```python
from build123d import *

# Parameters (mm, degrees)
SKETCH1_W           = 12.94
SKETCH1_H           = 7.76
BOSS_EXTRUDE1_DEPTH = 9.46
SKETCH2_R           = 2.87
BOSS_EXTRUDE2_DEPTH = 8.11
SKETCH4_W           = 0.73
SKETCH4_H           = 2.27
BOSS_EXTRUDE3_DEPTH = 4.33
BOSS_EXTRUDE4_DEPTH = 1.68
SKETCH6_R           = 6
BOSS_EXTRUDE5_DEPTH = 1.7
BOSS_EXTRUDE6_DEPTH = 1.68


with BuildPart() as part:
    # Sketch1 → Boss-Extrude1 (new body)
    with BuildSketch(Plane.XY):
        Rectangle(SKETCH1_W, SKETCH1_H)
    extrude(amount=BOSS_EXTRUDE1_DEPTH)

    # Sketch2 → Boss-Extrude2 (add)
    with BuildSketch(Plane.XY.offset(9.46)):
        Circle(SKETCH2_R)
    extrude(amount=BOSS_EXTRUDE2_DEPTH)

    # Sketch3 → Revolve1 (revolve)
    with BuildSketch(Plane(origin=(0, 0, 0), x_dir=(1, 0, 0), z_dir=(0, 1, 0))):
        with BuildLine():
            Line((0.46866366, -17.57), (-2.564053278, -27.111612822))
            ThreePointArc((-2.564053278, -27.111612822), (-3.316297804, -27.98726181), (-4.468815416, -28.053111116))
            Line((-4.468815416, -28.053111116), (-0.702418437, -17.57))
            Line((-0.702418437, -17.57), (0.46866366, -17.57))
        make_face()
    revolve(axis=Axis((-4.468815416, 0, 28.053111116), (0.3381215193488044, 0, -0.9411024589029912)))

    # Sketch4 → Boss-Extrude3 (add)
    with BuildSketch(Plane(origin=(0, 0, 0), x_dir=(-1, 0, 0), z_dir=(0, 0, -1))):
        Rectangle(SKETCH4_W, SKETCH4_H)
        with Locations((-4.475, 0)):
            Rectangle(SKETCH4_W, SKETCH4_H)
        with Locations((4.475, 0)):
            Rectangle(SKETCH4_W, SKETCH4_H)
    extrude(amount=BOSS_EXTRUDE3_DEPTH)

    # Sketch5 → Boss-Extrude4 (add)
    with BuildSketch(Plane.XY.offset(11.46)):
        Polygon((-2.309401077, -4), (2.309401077, -4), (4.618802154, 0), (2.309401077, 4), (-2.309401077, 4), (-4.618802154, 0), align=None)
    extrude(amount=-BOSS_EXTRUDE4_DEPTH)

    # Sketch6 → Boss-Extrude5 (add)
    with BuildSketch(Plane.XY.offset(13.46)):
        Circle(SKETCH6_R)
    extrude(amount=BOSS_EXTRUDE5_DEPTH)

    # Sketch7 → Boss-Extrude6 (add)
    with BuildSketch(Plane.XY.offset(15.16)):
        Polygon((-2.309401077, -4), (2.309401077, -4), (4.618802154, 0), (2.309401077, 4), (-2.309401077, 4), (-4.618802154, 0), align=None)
    extrude(amount=BOSS_EXTRUDE6_DEPTH)


solid = part.part
```
The model under review builds one solid part; all positions refer to its coordinate system, in mm. A direction names the side the tool comes from. Coordinates: 2 decimals unless noted, no trailing zeros. Write each loop counter-clockwise with the first axis right and the second up, starting at its lowest first coordinate (ties: lowest second). Pieces come first, ordered by that corner, then holes. Notation, with made-up numbers: (25.25, 40) - (62.25, 40) arc R23 cw to (62.25, 62) - close; hole circle Ø8 at (66.25, -14). An arc over 180 degrees is marked (long way). Answer in a Markdown table with one row per item. Add a question column.
Q1. Clearance check with flat-ended pins moving along their axes: pin 1 (2 mm diameter, centred on x = 4, y = -3, fed in from +Z); pin 2 (0.8 mm diameter, centred on x = 0.5, z = 10.5, fed in from -Y); pin 3 (1.8 mm diameter, centred on y = 0.5, z = -3, fed in from +X). State where each tip first meets the part, or that it passes through.
Q2. To check wall thickness, follow line 1 along Z through (x, y) = (0.5, -3); line 2 along Z through (x, y) = (4.75, 2); line 3 along Z through (x, y) = (-2, -1.5). State the ranges of each line that lie inside material, in increasing order. Write a range as from..to.
Q3. For faces 3 (the face through (4.11, 0, -2)), 4 (the face through (-2, 3, 9.46)), 5 (the face through (0, 4, 11)), 6 (the face through (3.448, -2.028, 15.988)), list the 3-axis set-ups (+Z, -Z, +X, -X, +Y, -Y) from which the entire face can be reached by the end or side of a thin tool; tool diameter is ignored.
Q4. Consider section A-A on x = 3.75. Give the boundary of the cut face in (y, z).
Q5. Consider section C-C on z = 8. Give the boundary of the cut face in (x, y), then the cut area to 3 significant figures.
Q6. Draft analysis for pull direction Z (two halves, no side actions). For faces 1 (the face through (-4.84, 0, -2)), 2 (the face through (-3.48, -1.97, 10.63)), state which applies: +Z half, -Z half, draft (parallel to the pull), parting line (faces both ways), or undercut.
Q7. Consider section B-B on z = 13. Give the boundary of the cut face in (x, y).
Answers below:
| question | item | result |
|---|---|---|
| 1 | pin 1 | z = 16.84 |
| 1 | pin 2 | y = -4 |
| 1 | pin 3 | x = 4.84 |
| 2 | line 1 | 0..9.46, 9.78..11.46, 13.46..16.84 |
| 2 | line 2 | 0..9.46, 13.46..15.16 |
| 2 | line 3 | 0..17.57 |
| 3 | face 3 | -Z, +Y, -Y |
| 3 | face 4 | none |
| 3 | face 5 | -Z, +X, -X, +Y |
| 3 | face 6 | +Z, +X, -Y |
| 4 | outline | (-4.68, 13.46) - (4.68, 13.46) - (4.68, 15.16) - (1.5, 15.16) - (1.5, 16.84) - (-1.5, 16.84) - (-1.5, 15.16) - (-4.68, 15.16) - close; (-3.88, 0) - (3.88, 0) - (3.88, 9.46) - (-3.88, 9.46) - close; (-1.5, 9.78) - (1.5, 9.78) - (1.5, 11.46) - (-1.5, 11.46) - close |
| 5 | outline | (-6.47, -3.88) - (6.47, -3.88) - (6.47, 3.88) - (-6.47, 3.88) - close |
| 5 | area | 100 mm² |
| 6 | face 1 | draft |
| 6 | face 2 | undercut |
| 7 | outline | circle Ø5.74 at (0, 0) |
